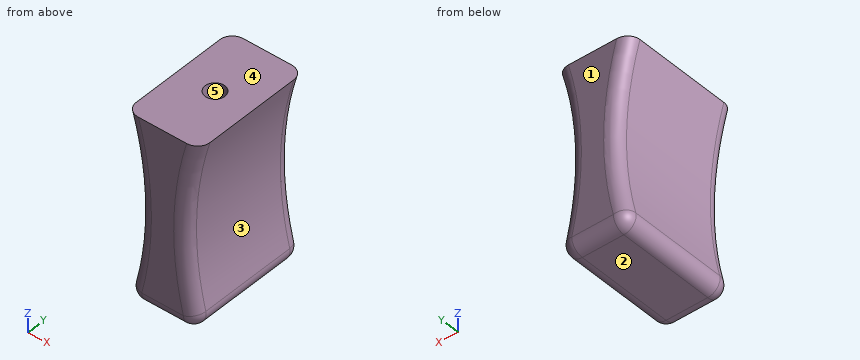
```python
from build123d import *

# Parameters (mm, degrees)
F1_DEPTH = 6.35
F2_R     = 1.016
F3_DEPTH = 15.875
F4_R     = 1.27


with BuildPart() as f1:
    # F0 (on Front) → F1 (new body, symmetric)
    with BuildSketch(Plane.XZ):
        with BuildLine():
            Line((0, 0), (3.81, 0))
            ThreePointArc((3.81, 0), (2.422893, 9.525), (3.81, 19.05))
            Line((3.81, 19.05), (0, 19.05))
            Line((0, 19.05), (0, 0))
        make_face()
        with BuildLine():
            Line((-3.81, 0), (0, 0))
            Line((0, 0), (0, 19.05))
            Line((0, 19.05), (-3.81, 19.05))
            ThreePointArc((-3.81, 19.05), (-2.422893, 9.525), (-3.81, 0))
        make_face()
    extrude(amount=F1_DEPTH, both=True)

    # F2 (on face) → F3 (cut)
    with BuildSketch(Plane.XY.offset(19.05)):
        Circle(F2_R)
    extrude(amount=-F3_DEPTH, mode=Mode.SUBTRACT)

    # F4
    f4_edges = [f1.edges().sort_by_distance(p)[0] for p in [
        (2.422893, -6.35, 9.525),
        (-2.422893, -6.35, 9.525),
        (0, -6.35, 0),
        (3.81, 0, 0),
        (0, 6.35, 0),
        (-3.81, 0, 0),
        (-2.422893, 6.35, 9.525),
        (2.422893, 6.35, 9.525),
    ]]
    fillet(f4_edges, radius=F4_R)


solid = f1.part
```
Part model, mm, in its own coordinate system. Face numbers are marked on the shaded views. A direction names the side the tool comes from. Round coordinates to 2 decimals unless told otherwise and drop trailing zeros. Order: outer loops, then holes, each group sorted by start corner. A loop starts at its lowest first (then second) coordinate and runs counter-clockwise, first axis right, second up. Notation, with made-up numbers: M -13.5,46 L 21.5,46 A30 cw 21.5,82 Z; hole C 8.25,-39 d6. An arc over 180 degrees is marked long. Answer in a Markdown table with one row per item. Add a question column.
Q1. Pin check, flat tips, straight feed: pin 1 (1 mm diameter, centred on x = -2, z = 11, fed in from -Y); pin 2 (5 mm diameter, centred on y = 0, z = 11, fed in from +X); pin 3 (6 mm diameter, centred on y = 0.5, z = 14, fed in from -X). Stop position of each tip, or through.
Q2. 3-axis set-ups, long thin cutter, end or side, ignore diameter. For the marked faces 4 and 5: which of +Z, -Z, +X, -X, +Y, -Y reach the whole face in a straight line?
Q3. Cut at A-A on x = 0. Give the cut face in (y, z) (3 decimals).
Q4. Cut at B-B on y = -0.25. Give the cut face in (x, z) (3 decimals).
Q5. Wall check: L1, parallel to Y at x = 0, z = 5; L2, parallel to X at y = -2, z = 1.25; L3, parallel to X at y = 3.5, z = 7.5. Give the ranges that are in metal, low to high. Write a range as from..to.
Q6. Mould opens along Z. For the marked faces 1, 2 and 3 say: +Z half, -Z half, draft (parallel to the pull), parting line (faces both ways), or undercut.
Q7. Cut at C-C on y = -4. Give the cut face in (x, z) (3 decimals).
Established:
| question | item | result |
|---|---|---|
| 1 | pin 1 | stops at y = -6.31 |
| 1 | pin 2 | stops at x = 2.66 |
| 1 | pin 3 | stops at x = -3.27 |
| 2 | face 4 | +Z, +X, -X, +Y, -Y |
| 2 | face 5 | +Z |
| 3 | outline | M -6.35,1.27 A1.27 ccw -5.08,0 L 5.08,0 A1.27 ccw 6.35,1.27 L 6.35,19.05 L 1.016,19.05 L 1.016,3.175 L -1.016,3.175 L -1.016,19.05 L -6.35,19.05 Z |
| 4 | outline | M -3.81,19.05 A33.397 cw -3.384,1.572 A1.27 ccw -2.15,0 L 2.15,0 A1.27 ccw 3.384,1.572 A33.397 cw 3.81,19.05 L 0.985,19.05 L 0.985,3.175 L -0.985,3.175 L -0.985,19.05 Z |
| 5 | L1 | y = -6.35..-1.02, 1.02..6.35 |
| 5 | L2 | x = -3.42..3.42 |
| 5 | L3 | x = -2.48..2.48 |
| 6 | face 1 | draft |
| 6 | face 2 | -Z half |
| 6 | face 3 | undercut |
| 7 | outline | M -3.81,19.05 A33.397 cw -3.384,1.572 A1.27 ccw -2.15,0 L 2.15,0 A1.27 ccw 3.384,1.572 A33.397 cw 3.81,19.05 Z |
